Autodesk Inventor part; units mm, degrees
ref_plane "YZ Plane" through (0, 0, 0) normal (1, 0, 0) x (0, 1, 0)
ref_plane "XZ Plane" through (0, 0, 0) normal (0, 1, 0) x (-1, 0, 0)
ref_plane "XY Plane" through (0, 0, 0) normal (0, 0, 1) x (1, 0, 0)
sketch "Sketch1" plane through (0, 0, 0) normal (0, 1, 0) x (-1, 0, 0)
  line L0 (9.278, 4.7758) -> (9.278, -28.2242)
  line L1 (9.278, -28.2242) -> (47.278, -28.2242)
  line L2 (47.278, -28.2242) -> (47.278, -22.2242)
  line L3 (47.278, -22.2242) -> (55.278, -22.2242)
  line L4 (55.278, -22.2242) -> (55.278, -28.2242)
  line L5 (55.278, 135.7758) -> (55.278, 129.7758)
  line L6 (55.278, 129.7758) -> (47.278, 129.7758)
  line L7 (47.278, 129.7758) -> (47.278, 135.7758)
  line L8 (47.278, 135.7758) -> (9.278, 135.7758)
  line L9 (9.278, 135.7758) -> (9.278, 102.7758)
  line L10 (9.278, 4.7758) -> (9.278, 4.7758)
  line L11 (9.278, 4.7758) -> (9.278, 102.7758)
  line L12 (9.278, 102.7758) -> (9.278, 102.7758)
  line L13 (54.278, 130.7758) -> (54.278, 136.7758)
  line L14 (8.278, 136.7758) -> (94.278, 136.7758)
  line L15 (94.278, -29.2242) -> (8.278, -29.2242)
  line L16 (54.278, -29.2242) -> (54.278, -23.2242)
  line L17 (54.278, -23.2242) -> (48.278, -23.2242)
  line L18 (48.278, -23.2242) -> (48.278, -29.2242)
  line L19 (8.278, -29.2242) -> (8.278, 3.7758)
  line L20 (8.278, 103.7758) -> (8.278, 136.7758)
  line L21 (48.278, 136.7758) -> (48.278, 130.7758)
  line L22 (8.278, 103.7758) -> (8.278, 3.7758)
  line L23 (54.278, 130.7758) -> (48.278, 130.7758)
  line L24 (94.278, -29.2242) -> (94.278, 136.7758)
  line L25 (55.278, 135.7758) -> (94.278, 135.7758)
  line L26 (55.278, -28.2242) -> (94.278, -28.2242)
  line L27 (94.278, 135.7758) -> (93.278, 135.7758)
  line L28 (93.278, 135.7758) -> (93.278, -28.2242)
  line L29 (93.278, -28.2242) -> (94.278, -28.2242)
  line L30 (94.278, -28.2242) -> (94.278, 135.7758)
  line L31 (8.278, 3.7758) -> (8.278, 3.7758)
  line L32 (8.278, 103.7758) -> (8.278, 103.7758)
  point P0 (0, 0)
  point P1 (0, 0)
  dimension "d0" = 1
  dimension "d4" = 1
  dimension "d5" = 1
  dimension "d6" = 1
  dimension "d7" = 1
  dimension "d10" = 1
  dimension "d12" = 1
  dimension "d13" = 1
  dimension "d14" = 1
  dimension "d15" = 1
  dimension "d16" = 6
  dimension "d17" = 0
  dimension "d18" = 0
  dimension "d25" = 1
  dimension "d75" = 164
  dimension "d76" = 164
  dimension "d77" = 166
  dimension "d79" = 33
  dimension "d82" = 33
  dimension "d95" = 0
  dimension "d96" = 86
  dimension "d97" = 1
  dimension "d98" = 86
extrude "Extrusion2" add sketch "Sketch1" along normal blind 2 contours L11 L9 L8 L7 L6 L5 L25 L28 L26 L4 L3 L2 L1 L0
sketch "Sketch2" plane through (0, 2, 0) normal (0, 1, 0) x (1, 0, 0)
  circle A0 centre (-12.278, 25.2242) radius 1.5
  line L0 (-9.278, -135.7758) -> (-9.278, 28.2242)
  line L1 (-9.278, 28.2242) -> (-47.278, 28.2242)
  line L2 (-47.278, 22.2242) -> (-55.278, 22.2242)
  line L3 (-51.278, 22.2242) -> (-51.278, -30.1136)
  circle A1 centre (-90.278, 25.2242) radius 1.5
  line L4 (-9.278, -135.7758) -> (-9.278, 28.2242)
  line L5 (-9.278, -53.7758) -> (-80.3163, -53.7758)
  circle A2 centre (-12.278, -132.7758) radius 1.5
  circle A3 centre (-90.278, -132.7758) radius 1.5
  point P0 (0, 0)
  point P1 (-49.278, -4.7758)
  point P2 (-9.278, -102.7758)
  point P3 (-9.278, -4.7758)
  dimension "d26" = 3
  dimension "d27" = 3
  dimension "d28" = 3
extrude "Extrusion3" cut sketch "Sketch2" against normal blind 10
sketch "Sketch3" plane through (0, 2, 0) normal (0, 1, 0) x (1, 0, 0)
  circle A0 centre (-36.278, -67.7758) radius 1.25
  circle A1 centre (-36.278, -67.7758) radius 1.25
  circle A2 centre (-36.278, -125.7758) radius 1.25
  circle A3 centre (-36.278, -125.7758) radius 1.25
  circle A4 centre (-85.278, -67.7758) radius 1.25
  circle A5 centre (-85.278, -67.7758) radius 1.25
  circle A6 centre (-85.278, -125.7758) radius 1.25
  circle A7 centre (-85.278, -125.7758) radius 1.25
  line L0 (-47.278, -135.7758) -> (-9.278, -135.7758)
  line L1 (-93.278, 28.2242) -> (-93.278, -135.7758)
  circle A8 centre (-36.278, -67.7758) radius 3
  circle A9 centre (-36.278, -125.7758) radius 3
  circle A10 centre (-85.278, -67.7758) radius 3
  circle A11 centre (-85.278, -125.7758) radius 3
  point P0 (0, 0)
  point P1 (40, -28)
  dimension "d31" = 49
  dimension "d32" = 58
  dimension "d33" = 49
  dimension "d34" = 58
  dimension "d35" = 10
  dimension "d36" = 10
  dimension "d37" = 8
  dimension "d38" = 8
  dimension "d70" = 6
  dimension "d71" = 6
  dimension "d72" = 6
  dimension "d73" = 6
extrude "Extrusion4" add sketch "Sketch3" along normal blind 7
sketch "Sketch6" plane through (0, 2, 0) normal (0, 1, 0) x (1, 0, 0)
  line L0 (-93.278, 28.2242) -> (-93.278, -135.7758)
  line L1 (-93.278, 28.2242) -> (-93.278, 21.2242)
  line L2 (-93.278, 21.2242) -> (-89.278, 21.2242)
  line L3 (-89.278, 21.2242) -> (-89.278, 12.2242)
  line L4 (-89.278, 12.2242) -> (-93.278, 12.2242)
  line L5 (-93.278, 21.2242) -> (-93.278, 12.2242)
  line L6 (-93.278, -135.7758) -> (-93.278, -128.7758)
  line L7 (-93.278, -128.7758) -> (-89.278, -128.7758)
  line L8 (-89.278, -128.7758) -> (-89.278, -119.7758)
  line L9 (-89.278, -119.7758) -> (-93.278, -119.7758)
  line L10 (-93.278, -128.7758) -> (-93.278, -119.7758)
  point P0 (0, 0)
  dimension "d63" = 7
  dimension "d64" = 4
  dimension "d65" = 9
  dimension "d66" = 7
  dimension "d67" = 9
  dimension "d83" = 4
extrude "Extrusion7" cut sketch "Sketch6" against normal blind 10
sketch "Sketch7" plane through (0, 2, 0) normal (0, 1, 0) x (1, 0, 0)
  line L0 (-9.278, -135.7758) -> (-9.278, 28.2242)
  line L1 (-9.278, 28.2242) -> (-47.278, 28.2242)
  line L2 (-47.278, 28.2242) -> (-47.278, 22.2242)
  line L3 (-9.278, -135.7758) -> (-9.278, 28.2242)
  line L4 (-9.278, -4.7758) -> (-49.278, -4.7758)
  line L5 (-49.278, -102.7758) -> (-9.278, -102.7758)
  line L6 (-47.278, 28.2242) -> (-47.278, 13.2242)
  line L7 (-47.278, 13.2242) -> (-17.278, 13.2242)
  line L8 (-17.278, 13.2242) -> (-17.278, 28.2242)
  line L9 (-9.278, 28.2242) -> (-47.278, 28.2242)
  point P0 (0, 0)
  dimension "d94" = 15
extrude "Extrusion8" cut sketch "Sketch7" against normal blind 10
chamfer "Chamfer1" distance 2 angle 45 4 edges at (-88.278, 2, 67.7758) (-39.278, 2, 125.7758) (-39.278, 2, 67.7758) (-88.278, 2, 125.7758)
equation "\"d36\" = d35"
equation "\"d38\" = d37"
CAD build for the part. Positions are in the model's coordinates, mm. A direction names the side the tool comes from. Give positions to 0.01 mm unless a question says otherwise; leave off trailing zeros. Write each loop counter-clockwise with the first axis right and the second up, starting at its lowest first coordinate (ties: lowest second). Pieces come first, ordered by that corner, then holes. Notation, with made-up numbers: (5, 66) -> (14, 66) arc R17 cw to (14, 78) -> close; hole circle Ø1 at (13.25, -33.5). An arc over 180 degrees is marked (long way). Return JSON: item names as keys, results as strings.
Item 1: Band-saw the part on C-C (z = 8.5). List the corners of the cut face in (x, y).
Answer below:
{"outline": "(-93.28, 0) -> (-9.28, 0) -> (-9.28, 2) -> (-93.28, 2) -> close"}
Item 2: Band-saw the part on B-B (x = -70). List the corners of the cut face in (y, z).
Answer below:
{"outline": "(0, -28.22) -> (2, -28.22) -> (2, 135.78) -> (0, 135.78) -> close"}
Item 3: Drop flat-ended pins along their axis: pin 1 (1.5 mm diameter, centred on x = -36, z = -9, fed in from +Y); pin 2 (2 mm diameter, centred on y = 0.5, z = -17.5, fed in from -X). Give the stop position or say it passes through.
Answer below:
{"pin 1": "stops at y = 2", "pin 2": "stops at x = -89.28"}
Item 4: Two-plate mould, pull along Z, no slides. Class faces 4 (the cylindrical face through (-33.417, 6.465, 68.677)), 5 (the flat face through (-35, 9, 126.4)): +Z half, -Z half, draft (parallel to the pull), parting line (faces both ways), or undercut.
Answer below:
{"face 4": "undercut", "face 5": "draft"}
Item 5: Tool access for faces 1 (the cylindrical face through (-34.67, 6.46, 128.31)), 2 (the flat face through (-89.278, 1, 124)), 3 (the cylindrical face through (-91.468, 1.014, 133.689)): list every direction of +Z, -Z, +X, -X, +Y, -Y with a clear straight run to the whole face (end or side of a thin tool).
Answer below:
{"face 1": "+Y", "face 2": "-X, +Y, -Y", "face 3": "+Y, -Y"}
Item 6: Drill centre lines: probe 1 along Y at (x, z) = (-73.5, 87); probe 2 along Z at (x, y) = (-37, 6); probe 3 along Y at (x, z) = (-33, 129). Where is each one in solid material? Low to high.
Answer below:
{"probe 1": "y = 0 to 2", "probe 2": "z = 64.86 to 66.76, 68.8 to 70.69, 122.86 to 124.76, 126.8 to 128.69", "probe 3": "y = 0 to 2.4"}
Item 7: Band-saw the part on A-A (y = 5.5). List the corners of the cut face in (x, z).
Answer below:
{"outline": "circle Ø6 at (-85.28, 67.78); circle Ø6 at (-85.28, 125.78); circle Ø6 at (-36.28, 67.78); circle Ø6 at (-36.28, 125.78); hole circle Ø2.5 at (-85.28, 67.78); hole circle Ø2.5 at (-85.28, 125.78); hole circle Ø2.5 at (-36.28, 67.78); hole circle Ø2.5 at (-36.28, 125.78)"}
